Part model, mm, in its own coordinate system. A direction names the side the tool comes from. Give positions to 0.01 mm unless a question says otherwise; leave off trailing zeros. Write each loop counter-clockwise with the first axis right and the second up, starting at its lowest first coordinate (ties: lowest second). Pieces come first, ordered by that corner, then holes.
from build123d import *

# Parameters (mm, degrees)
REVOLVE1_ANGLE      = 180
SKETCH4_R           = 50
BOSS_EXTRUDE1_DEPTH = 7
SKETCH5_R           = 34.5
BOSS_EXTRUDE2_DEPTH = 12
SKETCH6_R           = 39
BOSS_EXTRUDE4_DEPTH = 4
SKETCH7_R           = 30
CUT_EXTRUDE1_DEPTH  = 24
CUT_EXTRUDE2_DEPTH  = 10


with BuildPart() as part:
    # Sketch1 → Revolve1 (revolve)
    with BuildSketch(Plane(origin=(0, 0, 0), x_dir=(1, 0, 0), z_dir=(0, 1, 0))):
        with BuildLine():
            Line((1.491717845, 54.979766986), (-1.491717845, -54.979766986))
            ThreePointArc((-1.491717845, -54.979766986), (54.979766986, -1.491717845), (1.491717845, 54.979766986))
        make_face()
    revolve(axis=Axis((1.491717845, 0, -54.979766986), (-0.027122143, 0, 0.999632127)), revolution_arc=REVOLVE1_ANGLE)

    # Sketch2 → Cut-Revolve1 (revolve, cut)
    with BuildSketch(Plane.XZ):
        with BuildLine():
            Line((49.980692072, 1.389395568), (-49.980692072, -1.389395568))
            ThreePointArc((-49.980692072, -1.389395568), (-1.389395568, 49.980692072), (49.980692072, 1.389395568))
        make_face()
    revolve(axis=Axis((49.980692072, 0, 1.389395568), (-0.999613841, 0, -0.027787911)), mode=Mode.SUBTRACT)

    # Sketch4 → Boss-Extrude1 (add)
    with BuildSketch(Plane.XZ):
        Circle(SKETCH4_R)
    extrude(amount=-BOSS_EXTRUDE1_DEPTH)

    # Sketch5 → Boss-Extrude2 (add)
    with BuildSketch(Plane.XZ):
        Circle(SKETCH5_R)
    extrude(amount=BOSS_EXTRUDE2_DEPTH)

    # Sketch6 → Boss-Extrude4 (add)
    with BuildSketch(Plane.XZ.offset(12)):
        Circle(SKETCH6_R)
    extrude(amount=-BOSS_EXTRUDE4_DEPTH)

    # Sketch7 → Cut-Extrude1 (cut)
    with BuildSketch(Plane.XZ.offset(12)):
        Circle(SKETCH7_R)
    extrude(amount=-CUT_EXTRUDE1_DEPTH, mode=Mode.SUBTRACT)

    # Sketch8 → Cut-Extrude2 (cut)
    with BuildSketch(Plane.XZ.offset(12)):
        with BuildLine():
            ThreePointArc((37.671107225, 10.093942759), (19.5, 33.774990748), (-10.093942759, 37.671107225))
            Line((-10.093942759, 37.671107225), (-9.058666579, 33.80740392))
            ThreePointArc((-9.058666579, 33.80740392), (17.5, 30.310889132), (33.80740392, 9.058666579))
            Line((33.80740392, 9.058666579), (37.671107225, 10.093942759))
        make_face()
        with BuildLine():
            ThreePointArc((-10.093942759, -37.671107225), (19.5, -33.774990748), (37.671107225, -10.093942759))
            Line((37.671107225, -10.093942759), (33.80740392, -9.058666579))
            ThreePointArc((33.80740392, -9.058666579), (17.5, -30.310889132), (-9.058666579, -33.80740392))
            Line((-9.058666579, -33.80740392), (-10.093942759, -37.671107225))
        make_face()
        with BuildLine():
            Line((-24.748737342, 24.748737342), (-27.577164466, 27.577164466))
            ThreePointArc((-27.577164466, 27.577164466), (-39, 0), (-27.577164466, -27.577164466))
            Line((-27.577164466, -27.577164466), (-24.748737342, -24.748737342))
            ThreePointArc((-24.748737342, -24.748737342), (-35, 0), (-24.748737342, 24.748737342))
        make_face()
    extrude(amount=-CUT_EXTRUDE2_DEPTH, mode=Mode.SUBTRACT)


solid = part.part
1) Saw through at D-D (x = -36.5). Write the cut outline in (y, z).
Check result:
outline: (0, -41.14) arc R41.14 ccw to (0, 41.14) - close; hole (7, -33.45) arc R34.17 ccw to (7, 33.45) - close
2) Saw through at A-A (x = 0). Write the cut outline in (y, z), and give its area (3 significant figures).
Check result:
outline: (-12, -35) - (-8, -35) - (-8, -34.5) - (0, -34.5) - (0, -55) arc R55 ccw to (0, 55) - (0, 34.5) - (-8, 34.5) - (-8, 35) - (-12, 35) - (-12, 30) - (7, 30) - (7, 49.51) arc R50 cw to (7, -49.51) - (7, -30) - (-12, -30) - close
area: 1,210 mm2
3) Flat gauge pins, fed straight in: P1, Ø4, axis at x = 9.5, z = -20, coming from the -Y side; P2, Ø10, axis at x = -34, y = 15.5, coming from the +Z side; P3, Ø2, axis at x = 41, y = 32, coming from the -Z side. Where does each tip first touch, or does it go through?
Check result:
P1: stops at y = 43.79
P2: stops at z = 44.47
P3: stops at z = -20.57
4) Saw through at C-C (y = 29). Write the cut outline in (x, z), and give its area (3 significant figures).
Check result:
outline: circle Ø93.47 at (0, 0); hole circle Ø81.46 at (0, 0)
area: 1,650 mm2
5) Drill centre lines: L1, parallel to Z at x = 0, y = -6.5; L2, parallel to X at y = 24, z = -16.5; L3, parallel to X at y = 1, z = 19. Where is each one in solid material? Low to high.
Check result:
L1: z = -34.5 to -30, 30 to 34.5
L2: x = -46.66 to -40.64, 40.64 to 46.66
L3: x = -51.6 to -23.22, 23.22 to 51.6
6) Mould opens along Y. For faces 1 (the cylindrical face through (17.17, -10.03, 30.5)), 2 (the flat face through (-12, -12, -28)), 3 (the flat face through (-1, 7, -32)) say: +Y half, -Y half, draft (parallel to the pull), parting line (faces both ways), or undercut.
Check result:
face 1: draft
face 2: -Y half
face 3: undercut
7) 3-axis set-ups, long thin cutter, end or side, ignore diameter. For faces 4 (the flat face through (35, -8, 0)), 5 (the flat face through (-26, -10, -26)), 6 (the cylindrical face through (-19.624, -10.028, -33.703)): which of +Z, -Z, +X, -X, +Y, -Y reach the whole face in a straight line?
Check result:
face 4: none
face 5: -X, -Y
face 6: -Z, -X, -Y
8) Saw through at B-B (z = 0). Write the cut outline in (x, y), and give its area (3 significant figures).
Check result:
outline: (-55, 0) - (-34.5, 0) - (-34.5, -8) - (-35, -8) - (-35, -12) - (-30, -12) - (-30, 7) - (-49.51, 7) arc R50 cw to (49.51, 7) - (30, 7) - (30, -12) - (39, -12) - (39, -8) - (34.5, -8) - (34.5, 0) - (55, 0) arc R55 ccw to start
area: 1,230 mm2
